Part model, mm, in its own coordinate system. A direction names the side the tool comes from. Give positions to 0.01 mm unless a question says otherwise; leave off trailing zeros. Write each loop counter-clockwise with the first axis right and the second up, starting at its lowest first coordinate (ties: lowest second). Pieces come first, ordered by that corner, then holes.
```python
from build123d import *

# Parameters (mm, degrees)
F0_W     = 96
F0_H     = 161.5
F1_DEPTH = 59
F2_T     = -2
F3_R     = 4
F4_DEPTH = 51
F6_D     = 16
F6_DEPTH = 3


with BuildPart() as f1:
    # F0 (on Top) → F1 (new body)
    with BuildSketch(Plane.XY):
        Rectangle(F0_W, F0_H)
    extrude(amount=F1_DEPTH)

    # F2
    f2_openings = [f1.faces().sort_by_distance(p)[0] for p in [
        (0, 0, 59),
    ]]
    offset(amount=F2_T, openings=f2_openings)

    # F3 (on face) → F4 (join)
    with BuildSketch(Plane.XY.offset(2)):
        with Locations((-41, 73.75)):
            Circle(F3_R)
        with Locations((41, 73.75)):
            Circle(F3_R)
        with Locations((41, -73.75)):
            Circle(F3_R)
        with Locations((-41, -73.75)):
            Circle(F3_R)
    extrude(amount=F4_DEPTH)

    # F6
    with Locations(Plane.YZ.offset(48)):
        with Locations((30.75, 27)):
            Hole(F6_D / 2, depth=F6_DEPTH)


solid = f1.part
```
1) Saw through at C-C, the plane y = 29. Write the cut outline in (x, z).
Answers follow:
outline: (-48, 0) - (48, 0) - (48, 19.19) - (46, 19.19) - (46, 2) - (-46, 2) - (-46, 59) - (-48, 59) - close; (46, 34.81) - (48, 34.81) - (48, 59) - (46, 59) - close
2) 3-axis set-ups, long thin cutter, end or side, ignore diameter. For faces 4 (the face through (40.133, 69.845, 27.143)), 5 (the face through (48, -1, 29)): which of +Z, -Z, +X, -X, +Y, -Y reach the whole face in a straight line?
Answers follow:
face 4: +Z
face 5: +Z, -Z, +X, +Y, -Y
3) Saw through at A-A, the plane z = 27. Write the cut outline in (x, y).
Answers follow:
outline: (-48, -80.75) - (48, -80.75) - (48, 22.75) - (46, 22.75) - (46, -78.75) - (-46, -78.75) - (-46, 78.75) - (46, 78.75) - (46, 38.75) - (48, 38.75) - (48, 80.75) - (-48, 80.75) - close; circle Ø8 at (-41, -73.75); circle Ø8 at (-41, 73.75); circle Ø8 at (41, -73.75); circle Ø8 at (41, 73.75)
4) Pin check, flat tips, straight feed: pin 1 Ø2 at (x, y) = (12.5, 40.5) entering from +Z; pin 2 Ø6.5 at (x, y) = (-42.5, 72.5) entering from +Z. Stop position of each tip, or through.
Answers follow:
pin 1: stops at z = 2
pin 2: stops at z = 53
5) Saw through at B-B, the plane z = 37.5. Write the cut outline in (x, y).
Answers follow:
outline: (-48, -80.75) - (48, -80.75) - (48, 80.75) - (-48, 80.75) - close; circle Ø8 at (-41, -73.75); circle Ø8 at (-41, 73.75); circle Ø8 at (41, -73.75); circle Ø8 at (41, 73.75); hole (-46, -78.75) - (46, -78.75) - (46, 78.75) - (-46, 78.75) - close
6) Wall check: L1, parallel to X at y = -33, z = 15.5; L2, parallel to Y at x = 25, z = 34; L3, parallel to Z at x = 47, y = 30. Give the ranges that are in metal, low to high.
Answers follow:
L1: x = -48 to -46, 46 to 48
L2: y = -80.75 to -78.75, 78.75 to 80.75
L3: z = 0 to 19.04, 34.96 to 59
7) Saw through at D-D, the plane x = 16. Write the cut outline in (y, z), then the cut area to 3 significant figures.
Answers follow:
outline: (-80.75, 0) - (80.75, 0) - (80.75, 59) - (78.75, 59) - (78.75, 2) - (-78.75, 2) - (-78.75, 59) - (-80.75, 59) - close
area: 551 mm2
8) Two-plate mould, pull along Y, no slides. Class faces 1 (the face through (-1, 80.75, 29)), 2 (the face through (-1, 1, 0)), 3 (the face through (-46, -1, 30)): +Y half, -Y half, draft (parallel to the pull), parting line (faces both ways), or undercut.
Answers follow:
face 1: +Y half
face 2: draft
face 3: undercut
